Read the model definition and answer for the solid it produces. Units are mm, in the model's axes. A direction names the side the tool comes from. Coordinates: 2 decimals unless noted, no trailing zeros. Write each loop counter-clockwise with the first axis right and the second up, starting at its lowest first coordinate (ties: lowest second). Pieces come first, ordered by that corner, then holes.
from build123d import *

# Parameters (mm, degrees)
SKETCH1_W           = 128.5875
SKETCH1_H           = 144.4625
BOSS_EXTRUDE1_DEPTH = 61.07176
SHELL1_T            = 6.35


with BuildPart() as part:
    # Sketch1 → Boss-Extrude1 (new body)
    with BuildSketch(Plane.XY):
        Rectangle(SKETCH1_W, SKETCH1_H)
    extrude(amount=-BOSS_EXTRUDE1_DEPTH)

    # Shell1
    shell1_openings = [part.faces().sort_by_distance(p)[0] for p in [
        (0, 0, -61.07176),
    ]]
    offset(amount=SHELL1_T, openings=shell1_openings, kind=Kind.INTERSECTION)


solid = part.part
Item 1: For faces 4 (the flat face through (-68, 0, -61.072)), 5 (the flat face through (-64.294, -1, -30)), determine the directions among +Z, -Z, +X, -X, +Y, -Y from which every point of the face is accessible in a straight line to the end or side of a thin tool.
Item 2: The part is cut by section B-B (y = 6). Give the vertices of the cut face in (x, z), and give its area (3 significant figures).
Item 3: Determine the mould class of faces 1 (the flat face through (-1, 72.231, -30)), 2 (the flat face through (-1, -78.581, -27)), 3 (the flat face through (70.644, -1, -27)) for opening direction X: +X half, -X half, draft (parallel to the pull), parting line (faces both ways), or undercut.
Item 4: The part is cut by section A-A (z = -46.5). Give the vertices of the cut face in (x, y).
Item 5: Given pin 1 (1 mm diameter, centred on x = 35, y = 37.5, fed in from -Z), flat-ended and moving along its own axis, determine where the tip first touches the part or whether it passes through.
Item 6: Find the intervals of material crossed by probe 1 along Y at (x, z) = (-59.5, -42); probe 2 along X at (y, z) = (5, -25); probe 3 along Z at (x, y) = (-27, -54.5), in increasing order.
Item 7: The part is cut by section C-C (x = 59). Give the vertices of the cut face in (y, z).
Answer:
1. face 4: -Z, +X, -X, +Y, -Y
1. face 5: -Z
2. outline: (-70.64, -61.07) - (-64.29, -61.07) - (-64.29, 0) - (64.29, 0) - (64.29, -61.07) - (70.64, -61.07) - (70.64, 6.35) - (-70.64, 6.35) - close
2. area: 1,670 mm2
3. face 1: undercut
3. face 2: draft
3. face 3: +X half
4. outline: (-70.64, -78.58) - (70.64, -78.58) - (70.64, 78.58) - (-70.64, 78.58) - close; hole (-64.29, -72.23) - (64.29, -72.23) - (64.29, 72.23) - (-64.29, 72.23) - close
5. pin 1: stops at z = 0
6. probe 1: y = -78.58 to -72.23, 72.23 to 78.58
6. probe 2: x = -70.64 to -64.29, 64.29 to 70.64
6. probe 3: z = 0 to 6.35
7. outline: (-78.58, -61.07) - (-72.23, -61.07) - (-72.23, 0) - (72.23, 0) - (72.23, -61.07) - (78.58, -61.07) - (78.58, 6.35) - (-78.58, 6.35) - close
